Read the model definition and answer for the solid it produces. Units are mm, in the model's axes. A direction names the side the tool comes from. Coordinates: 2 decimals unless noted, no trailing zeros. Loops run counter-clockwise (first coordinate to the right, second up) from the corner with the lowest first, then second, coordinate; pieces in that order, holes last. Notation, with made-up numbers: (38, 9.25) - (91, 9.25) arc R26 ccw to (91, 36.25) - close; hole circle Ø5 at (20.25, 47). An arc over 180 degrees is marked (long way). Use one line per item in the form item = value. Start each with the question number.
1) The mould has two halves that part along Z. Classify faces 1 (the face through (-4, 3, -32.333)), 2 (the face through (-4, 3, 28.667)), 3 (the face through (-4, 4, -2)): released by +Z, released by -Z, zero draft, split by the parting line, or undercut.
2) A cutting plane is placed at D-D (z = 0). Give the vertices of the cut face in (x, y), and give its area (3 significant figures).
3) A cutting plane is placed at A-A (z = 9.5). Give the vertices of the cut face in (x, y), and give its area (3 significant figures).
4) Each of these flat-tipped pins is pushed along its axis until it touches: P1, Ø1, axis at x = 3.5, y = 3, coming from the -Z side; P2, Ø11, axis at y = 10, z = -1.5, coming from the -X side; P3, Ø8, axis at x = 45, y = 13.5, coming from the +Z side. Where does it stop, or does it pass through?
5) Consider line 1 (Y direction, x = -26, z = 1); line 2 (Z direction, x = -27, y = 3); line 3 (X direction, y = 17.5, z = 1.5). Determine where each line is inside the solid, lowest interval first.
6) A cutting plane is placed at B-B (x = -24). Give the vertices of the cut face in (y, z).
7) A cutting plane is placed at C-C (y = 6.75). Give the vertices of the cut face in (x, z).
8) Which of the six approach directions +Z, -Z, +X, -X, +Y, -Y give full straight-line access (tool end or side, diameter ignored) to faces 4 (the face through (45, 14, -6.833)), 5 (the face through (40.045, 14, -2)), 6 (the face through (50.045, 10, -2)), 7 (the face through (45, 14, 3.167))?
from build123d import *

# Parameters (mm, degrees)
SKETCH1_W           = 110
SKETCH1_H           = 65
BOSS_EXTRUDE1_DEPTH = 2
SKETCH2_W           = 106
SKETCH2_H           = 61
BOSS_EXTRUDE3_DEPTH = 2
SKETCH6_W           = 10
SKETCH6_H           = 10
BOSS_EXTRUDE4_DEPTH = 19.5


with BuildPart() as part:
    # Sketch1 → Boss-Extrude1 (new body)
    with BuildSketch(Plane(origin=(0, 0, 0), x_dir=(1, 0, 0), z_dir=(0, 1, 0))):
        with Locations((-2.954873439, 1.833455829)):
            Rectangle(SKETCH1_W, SKETCH1_H)
    extrude(amount=BOSS_EXTRUDE1_DEPTH)

    # Sketch2 → Boss-Extrude3 (add)
    with BuildSketch(Plane(origin=(0, 2, 0), x_dir=(1, 0, 0), z_dir=(0, 1, 0))):
        with Locations((-2.954873439, 1.833455829)):
            Rectangle(SKETCH2_W, SKETCH2_H)
    extrude(amount=BOSS_EXTRUDE3_DEPTH)

    # Sketch6 → Boss-Extrude4 (add)
    with BuildSketch(Plane(origin=(0, 4, 0), x_dir=(1, 0, 0), z_dir=(0, 1, 0))):
        with Locations((45.045126561, 1.833455829)):
            Rectangle(SKETCH6_W, SKETCH6_H)
    extrude(amount=BOSS_EXTRUDE4_DEPTH)


solid = part.part
Found:
q1.face_1 = released by -Z
q1.face_2 = released by +Z
q1.face_3 = zero draft
q2.outline = (-57.95, 0) - (52.05, 0) - (52.05, 2) - (50.05, 2) - (50.05, 23.5) - (40.05, 23.5) - (40.05, 4) - (-55.95, 4) - (-55.95, 2) - (-57.95, 2) - close
q2.area = 627 mm^2
q3.outline = (-57.95, 0) - (52.05, 0) - (52.05, 2) - (50.05, 2) - (50.05, 4) - (-55.95, 4) - (-55.95, 2) - (-57.95, 2) - close
q3.area = 432 mm^2
q4.P1 = -32.33
q4.P2 = 40.05
q4.P3 = 3.17
q5.line_1 = 0 to 4
q5.line_2 = -32.33 to 28.67
q5.line_3 = 40.05 to 50.05
q6.outline = (0, -34.33) - (2, -34.33) - (2, -32.33) - (4, -32.33) - (4, 28.67) - (2, 28.67) - (2, 30.67) - (0, 30.67) - close
q7.outline = (40.05, -6.83) - (50.05, -6.83) - (50.05, 3.17) - (40.05, 3.17) - close
q8.face_4 = -Z, +X, -X, +Y
q8.face_5 = +Z, -Z, -X, +Y
q8.face_6 = +Z, -Z, +X, +Y
q8.face_7 = +Z, +X, -X, +Y
